Geometry: final body of the model. Coordinates: model frame, mm. A direction names the side the tool comes from. Give positions to 0.01 mm unless a question says otherwise; leave off trailing zeros. Order: outer loops, then holes, each group sorted by start corner. A loop starts at its lowest first (then second) coordinate and runs counter-clockwise, first axis right, second up. Notation, with made-up numbers: M 44,66.5 L 76,66.5 A12 cw 76,74.5 Z; hole C 78.25,-23 d8. An arc over 180 degrees is marked long. Write item = value, one per line. Start each with the question number.
from build123d import *

# Parameters (mm, degrees)
SKETCH1_W                    = 130
SKETCH1_H                    = 135
BASE_FLANGE2_DEPTH           = 1.5
EDGE_FLANGE5_STRIP_W         = 7.4732
EDGE_FLANGE5_STRIP_H         = 1.5
EDGE_FLANGE5_STRIP_CUT_DEPTH = 135
EDGE_FLANGE5_DEPTH           = 135
EDGE_FLANGE6_STRIP_W         = 7.4732
EDGE_FLANGE6_STRIP_H         = 1.5
EDGE_FLANGE6_STRIP_CUT_DEPTH = 135
EDGE_FLANGE6_DEPTH           = 135
EDGE_FLANGE7_STRIP_W         = 7.4732
EDGE_FLANGE7_STRIP_H         = 1.5
EDGE_FLANGE7_STRIP_CUT_DEPTH = 125.5268
EDGE_FLANGE7_DEPTH           = 125.5268
CUT_EXTRUDE1_START           = -130
CUT_EXTRUDE1_OUTLINE_R       = 4.25
CUT_EXTRUDE1_DEPTH           = 130
CUT_EXTRUDE1_START_2         = -127.7634
CUT_EXTRUDE1_2_DEPTH         = 125.5268
SKETCH39_R                   = 55
CUT_EXTRUDE2_DEPTH           = 10
EDGE_FLANGE8_STRIP_W         = 7.4732
EDGE_FLANGE8_STRIP_H         = 1.5
EDGE_FLANGE8_STRIP_CUT_DEPTH = 125.5268
EDGE_FLANGE8_DEPTH           = 125.5268


# Read off the part's stored shape, not the designer's step: Cut-Extrude1
# Sheet-metal steps are written as plain solids
with BuildPart() as part:
    # Sketch1 → Base-Flange2 (new body)
    with BuildSketch(Plane.XY):
        with Locations((1.766304348, -20.692934783)):
            Rectangle(SKETCH1_W, SKETCH1_H)
    extrude(amount=-BASE_FLANGE2_DEPTH)

    # Edge-Flange5 strip (across the edge) → Edge-Flange5 strip cut (cut)
    with BuildSketch(Plane(origin=(66.766304348, -88.192934783, 0), x_dir=(-1, 0, 0), z_dir=(0, 1, 0))):
        with Locations((-1.5, -0.75)):
            Rectangle(EDGE_FLANGE5_STRIP_W, EDGE_FLANGE5_STRIP_H)
    extrude(amount=EDGE_FLANGE5_STRIP_CUT_DEPTH, mode=Mode.SUBTRACT)

    # Edge-Flange5 section (across the edge) → Edge-Flange5 (add)
    with BuildSketch(Plane(origin=(66.766304348, -88.192934783, 0), x_dir=(-1, 0, 0), z_dir=(0, 1, 0))):
        with BuildLine():
            Line((0, 0.7366), (0, 63.5))
            Line((0, 63.5), (1.5, 63.5))
            Line((1.5, 63.5), (1.5, 0.7366))
            ThreePointArc((1.5, 0.7366), (1.715745145, 0.215745145), (2.2366, 0))
            Line((2.2366, 0), (2.2366, -1.5))
            ThreePointArc((2.2366, -1.5), (0.655084973, -0.844915027), (0, 0.7366))
        make_face()
    extrude(amount=EDGE_FLANGE5_DEPTH)

    # Edge-Flange6 strip (across the edge) → Edge-Flange6 strip cut (cut)
    with BuildSketch(Plane(origin=(-63.233695652, 46.807065217, 0), x_dir=(1, 0, 0), z_dir=(0, -1, 0))):
        with Locations((-1.5, -0.75)):
            Rectangle(EDGE_FLANGE6_STRIP_W, EDGE_FLANGE6_STRIP_H)
    extrude(amount=EDGE_FLANGE6_STRIP_CUT_DEPTH, mode=Mode.SUBTRACT)

    # Edge-Flange6 section (across the edge) → Edge-Flange6 (add)
    with BuildSketch(Plane(origin=(-63.233695652, 46.807065217, 0), x_dir=(1, 0, 0), z_dir=(0, -1, 0))):
        with BuildLine():
            Line((0, 0.7366), (0, 63.5))
            Line((0, 63.5), (1.5, 63.5))
            Line((1.5, 63.5), (1.5, 0.7366))
            ThreePointArc((1.5, 0.7366), (1.715745145, 0.215745145), (2.2366, 0))
            Line((2.2366, 0), (2.2366, -1.5))
            ThreePointArc((2.2366, -1.5), (0.655084973, -0.844915027), (0, 0.7366))
        make_face()
    extrude(amount=EDGE_FLANGE6_DEPTH)

    # Edge-Flange7 strip (across the edge) → Edge-Flange7 strip cut (cut)
    with BuildSketch(Plane(origin=(64.529704348, 46.807065217, 0), x_dir=(0, -1, 0), z_dir=(-1, 0, 0))):
        with Locations((-1.5, -0.75)):
            Rectangle(EDGE_FLANGE7_STRIP_W, EDGE_FLANGE7_STRIP_H)
    extrude(amount=EDGE_FLANGE7_STRIP_CUT_DEPTH, mode=Mode.SUBTRACT)

    # Edge-Flange7 section (across the edge) → Edge-Flange7 (add)
    with BuildSketch(Plane(origin=(64.529704348, 46.807065217, 0), x_dir=(0, -1, 0), z_dir=(-1, 0, 0))):
        with BuildLine():
            Line((0, 0.7366), (0, 22.5))
            Line((0, 22.5), (1.5, 22.5))
            Line((1.5, 22.5), (1.5, 0.7366))
            ThreePointArc((1.5, 0.7366), (1.715745145, 0.215745145), (2.2366, 0))
            Line((2.2366, 0), (2.2366, -1.5))
            ThreePointArc((2.2366, -1.5), (0.655084973, -0.844915027), (0, 0.7366))
        make_face()
    extrude(amount=EDGE_FLANGE7_DEPTH)

    # Cut-Extrude1 outline → Cut-Extrude1 (cut)
    with BuildSketch(Plane(origin=(66.766304348, 0, 0), x_dir=(0, 0, -1), z_dir=(1, 0, 0)).offset(CUT_EXTRUDE1_START)):
        with Locations((-14.5, -72.192934783)):
            Circle(CUT_EXTRUDE1_OUTLINE_R)
        Polygon((-17.5, 46.807065217), (-63.5, 46.807065217), (-63.5, -68.192934783), align=None)
    extrude(amount=CUT_EXTRUDE1_DEPTH, mode=Mode.SUBTRACT)

    # Cut-Extrude1 2 outline → Cut-Extrude1 2 (cut)
    with BuildSketch(Plane(origin=(66.766304348, 0, 0), x_dir=(0, 0, -1), z_dir=(1, 0, 0)).offset(CUT_EXTRUDE1_START_2)):
        Polygon((-17.5, 45.307065217), (-17.5, 46.807065217), (-18.1, 45.307065217), align=None)
    extrude(amount=CUT_EXTRUDE1_2_DEPTH, mode=Mode.SUBTRACT)

    # Sketch39 → Cut-Extrude2 (cut)
    with BuildSketch(Plane(origin=(0, 0, -1.5), x_dir=(-1, 0, 0), z_dir=(0, 0, -1))):
        with Locations((-1.766304348, -20.692934783)):
            Circle(SKETCH39_R)
    extrude(amount=-CUT_EXTRUDE2_DEPTH, mode=Mode.SUBTRACT)

    # Edge-Flange8 strip (across the edge) → Edge-Flange8 strip cut (cut)
    with BuildSketch(Plane(origin=(-60.997095652, -88.192934783, 0), x_dir=(0, 1, 0), z_dir=(1, 0, 0))):
        with Locations((-1.5, -0.75)):
            Rectangle(EDGE_FLANGE8_STRIP_W, EDGE_FLANGE8_STRIP_H)
    extrude(amount=EDGE_FLANGE8_STRIP_CUT_DEPTH, mode=Mode.SUBTRACT)

    # Edge-Flange8 section (across the edge) → Edge-Flange8 (add)
    with BuildSketch(Plane(origin=(-60.997095652, -88.192934783, 0), x_dir=(0, 1, 0), z_dir=(1, 0, 0))):
        with BuildLine():
            Line((0, 0.7366), (0, 63.5))
            Line((0, 63.5), (1.5, 63.5))
            Line((1.5, 63.5), (1.5, 0.7366))
            ThreePointArc((1.5, 0.7366), (1.715745145, 0.215745145), (2.2366, 0))
            Line((2.2366, 0), (2.2366, -1.5))
            ThreePointArc((2.2366, -1.5), (0.655084973, -0.844915027), (0, 0.7366))
        make_face()
    extrude(amount=EDGE_FLANGE8_DEPTH)


solid = part.part
1) Ray query, L1, parallel to Y at x = 66.25, z = 14.5; L2, parallel to Y at x = 23.5, z = 7.5; L3, parallel to X at y = -58.5, z = 8.5. Return the intervals inside material, ascending.
2) Cut plane C-C (y = -59.5). Return loops of the section in (x, z).
3) Draft query along Y for faces 1 (the cylindrical face through (66.006, -75.963, 12.539)), 2 (the flat face through (1, -86.693, 33)), 3 (the flat face through (-62.494, -11.498, 40.822)), 4 (the flat face through (1, -88.193, 32)). Return one class per face: pulls with the +Y half, pulls with the -Y half, needs draft (parallel to the pull), parting line crosses it, or undercut.
4) Pin query (flat end, axial travel): pin 1 Ø10 at (y, z) = (-72.19, 14.5) entering from -X; pin 2 Ø3 at (x, z) = (-17, 38) entering from +Y; pin 3 Ø1.7 at (y, z) = (-87.5, -1) entering from +X; pin 4 Ø1.6 at (x, y) = (-9.5, 46) entering from +Z. Return the tip coordinate at first contact, or that it passes through.
5) Cut plane D-D (x = 0.5). Return loops of the section in (y, z), plus the area to 3 significant figures.
6) Cut plane B-B (z = 6). Return loops of the section in (x, y), plus the area to 3 significant figures.
7) Access query for faces 5 (the flat face through (3, 45.307, 9)), 6 (the flat face through (3, 46.807, 9)), 7 (the flat face through (65.266, -37, 26)). Directions: +Z, -Z, +X, -X, +Y, -Y. A direction counts if a zero-diameter tool reaches every point of the face in a straight line with its end or side. Return the directions, or none.
8) Cut plane A-A (z = 14.5). Return loops of the section in (x, y).
Reply:
q1.L1 = -88.19 to -76.44, -67.94 to 46.81
q1.L2 = -88.19 to -86.69, 45.31 to 46.81
q1.L3 = -63.23 to -61.73, 65.27 to 66.77
q2.outline = M -63.23,0.74 A2.24 ccw -61,-1.5 L -37.21,-1.5 L -37.21,0 L -61,0 A0.74 cw -61.73,0.74 L -61.73,60.02 L -63.23,60.02 Z; M 40.74,-1.5 L 64.53,-1.5 A2.24 ccw 66.77,0.74 L 66.77,60.02 L 65.27,60.02 L 65.27,0.74 A0.74 cw 64.53,0 L 40.74,0 Z
q3.face_1 = undercut
q3.face_2 = undercut
q3.face_3 = pulls with the +Y half
q3.face_4 = pulls with the -Y half
q4.pin_1 = -63.23
q4.pin_2 = -86.69
q4.pin_3 = 66.58
q4.pin_4 = 17.5
q5.outline = M -88.19,0.74 A2.24 ccw -85.96,-1.5 L -75.68,-1.5 L -75.68,0 L -85.96,0 A0.74 cw -86.69,0.74 L -86.69,63.5 L -88.19,63.5 Z; M 34.29,-1.5 L 44.57,-1.5 A2.24 ccw 46.81,0.74 L 46.81,17.5 L 45.31,17.5 L 45.31,0.74 A0.74 cw 44.57,0 L 34.29,0 Z
q5.area = 157 mm²
q6.outline = M -63.23,-88.19 L -61.73,-88.19 L -61.73,46.81 L -63.23,46.81 Z; M -61,-88.19 L 64.53,-88.19 L 64.53,-86.69 L -61,-86.69 Z; M -61,45.31 L 64.53,45.31 L 64.53,46.81 L -61,46.81 Z; M 65.27,-88.19 L 66.77,-88.19 L 66.77,46.81 L 65.27,46.81 Z
q6.area = 782 mm²
q7.face_5 = +Z
q7.face_6 = +Z, -Z, +X, -X, +Y
q7.face_7 = +Z, +Y, -Y
q8.outline = M -63.23,-88.19 L -61.73,-88.19 L -61.73,-76.44 L -63.23,-76.44 Z; M -63.23,-67.94 L -61.73,-67.94 L -61.73,46.81 L -63.23,46.81 Z; M -61,-88.19 L 64.53,-88.19 L 64.53,-86.69 L -61,-86.69 Z; M -61,45.31 L 64.53,45.31 L 64.53,46.81 L -61,46.81 Z; M 65.27,-88.19 L 66.77,-88.19 L 66.77,-76.44 L 65.27,-76.44 Z; M 65.27,-67.94 L 66.77,-67.94 L 66.77,46.81 L 65.27,46.81 Z
